from build123d import *

# Parameters (mm, degrees)
ESBO_O1_W                          = 181
ESBO_O1_H                          = 77
RESSALTO_EXTRUS_O1_DEPTH           = 167
ESBO_O2_W                          = 181
ESBO_O2_H                          = 30
CORTE_EXTRUS_O1_DEPTH              = 10
ESBO_O3_R                          = 9
RESSALTO_EXTRUS_O2_DEPTH           = 20
RESSALTO_EXTRUS_O2_DRAFT           = 10
RESSALTO_EXTRUS_O2_PROFILE_2_DEPTH = 20
RESSALTO_EXTRUS_O2_PROFILE_2_DRAFT = 10


with BuildPart() as part:
    # Esboço1 → Ressalto-extrusão1 (new body)
    with BuildSketch(Plane(origin=(0, 0, 0), x_dir=(1, 0, 0), z_dir=(0, 1, 0))):
        with Locations((13.5, 6.669291339)):
            Rectangle(ESBO_O1_W, ESBO_O1_H)
    extrude(amount=RESSALTO_EXTRUS_O1_DEPTH)

    # Esboço2 → Corte-extrusão1 (cut)
    with BuildSketch(Plane(origin=(0, 167, 0), x_dir=(1, 0, 0), z_dir=(0, 1, 0))):
        with Locations((13.5, -16.830708661)):
            Rectangle(ESBO_O2_W, ESBO_O2_H)
    extrude(amount=-CORTE_EXTRUS_O1_DEPTH, mode=Mode.SUBTRACT)


with BuildPart() as ressalto_extrus_o2_tool:
    # Esboço3 → Ressalto-extrusão2 (with draft: the straight prism first)
    with BuildSketch(Plane(origin=(0, 157, 0), x_dir=(1, 0, 0), z_dir=(0, 1, 0))):
        with Locations((-61.5, -17.830708661)):
            Circle(ESBO_O3_R)
    extrude(amount=RESSALTO_EXTRUS_O2_DEPTH)
    # Ressalto-extrusão2: the draft: its side faces are tilted about the plane it starts from
    ressalto_extrus_o2_sides = [ressalto_extrus_o2_tool.faces().sort_by_distance(p)[0] for p in [
        (-70.5, 167, 17.830708661),
    ]]
    draft(ressalto_extrus_o2_sides, Plane(origin=(0, 157, 0), x_dir=(1, 0, 0), z_dir=(0, 1, 0)), RESSALTO_EXTRUS_O2_DRAFT)


with BuildPart() as part_1:
    add(part.part)

    # Ressalto-extrusão2: add ressalto_extrus_o2_tool
    add(ressalto_extrus_o2_tool.part)


with BuildPart() as ressalto_extrus_o2_profile_2_tool:
    # Esboço3 → Ressalto-extrusão2 profile 2 (with draft: the straight prism first)
    with BuildSketch(Plane(origin=(0, 157, 0), x_dir=(1, 0, 0), z_dir=(0, 1, 0))):
        with Locations((88.5, -17.830708661)):
            Circle(ESBO_O3_R)
    extrude(amount=RESSALTO_EXTRUS_O2_PROFILE_2_DEPTH)
    # Ressalto-extrusão2 profile 2: the draft: its side faces are tilted about the plane it starts from
    ressalto_extrus_o2_profile_2_sides = [ressalto_extrus_o2_profile_2_tool.faces().sort_by_distance(p)[0] for p in [
        (79.5, 167, 17.830708661),
    ]]
    draft(ressalto_extrus_o2_profile_2_sides, Plane(origin=(0, 157, 0), x_dir=(1, 0, 0), z_dir=(0, 1, 0)), RESSALTO_EXTRUS_O2_PROFILE_2_DRAFT)


with BuildPart() as part_2:
    add(part_1.part)

    # Ressalto-extrusão2 profile 2: add ressalto_extrus_o2_profile_2_tool
    add(ressalto_extrus_o2_profile_2_tool.part)


solid = part_2.part
Model file for the job. Use its own axes, mm. A direction names the side the tool comes from. Give positions to 0.01 mm unless a question says otherwise; leave off trailing zeros. Write each loop counter-clockwise with the first axis right and the second up, starting at its lowest first coordinate (ties: lowest second). Pieces come first, ordered by that corner, then holes. Notation, with made-up numbers: M 74.25,76 L 92.25,76 A25 cw 92.25,102 Z; hole C -17,-26.75 d3. An arc over 180 degrees is marked long. One line per item, written item: value. Start each with the question number.
Q1. Saw through at C-C, the plane x = 56. Write the cut outline in (y, z), plus the area to 3 significant figures.
Q2. 3-axis set-ups, long thin cutter, end or side, ignore diameter. For faces 4 (the flat face through (12, 162, 1.831)), 5 (the flat face through (12, 167, -22)), 6 (the flat face through (12, 0, -7)): which of +Z, -Z, +X, -X, +Y, -Y reach the whole face in a straight line?
Q3. Two-plate mould, pull along X, no slides. Class faces 1 (the flat face through (12, 82, -45.169)), 2 (the conical face through (91.67, 169.082, 23.925)), 3 (the flat face through (-77, 82, -6)): +X half, -X half, draft (parallel to the pull), parting line (faces both ways), or undercut.
Q4. Saw through at A-A, the plane x = 88.5. Write the cut outline in (y, z).
Q5. Saw through at B-B, the plane z = -21. Write the cut outline in (x, y), plus the area to 3 significant figures.
Q6. Drop flat-ended pins along their axis: pin 1 Ø3 at (x, z) = (24.5, -25.5) entering from +Y; pin 2 Ø11 at (x, y) = (0.5, 163.5) entering from +Z; pin 3 Ø15 at (x, z) = (46, 17.5) entering from +Y. Give the stop position or say it passes through.
Q7. Probe probe 1 along Y at (x, z) = (8, -1); probe 2 along Y at (x, z) = (37.5, 11.5); probe 3 along Z at (x, y) = (-20.5, 158.5). List the from-to ranges inside material, lowest first. Write a range as [from, to].
Output values:
1. outline: M 0,-45.17 L 167,-45.17 L 167,1.83 L 157,1.83 L 157,31.83 L 0,31.83 Z
1. area: 12,600 mm²
2. face 4: +X, -X, +Y
2. face 5: -Z, +X, -X, +Y
2. face 6: +Z, -Z, +X, -X, -Y
3. face 1: draft
3. face 2: undercut
3. face 3: -X half
4. outline: M 0,-45.17 L 167,-45.17 L 167,1.83 L 157,1.83 L 157,8.83 L 177,12.36 L 177,23.3 L 157,26.83 L 157,31.83 L 0,31.83 Z
5. outline: M -77,0 L 104,0 L 104,167 L -77,167 Z
5. area: 30,200 mm²
6. pin 1: stops at y = 167
6. pin 2: stops at z = 1.83
6. pin 3: stops at y = 157
7. probe 1: y = [0, 167]
7. probe 2: y = [0, 157]
7. probe 3: z = [-45.17, 1.83]
